```python
from build123d import *

# Parameters (mm, degrees)
CUT_EXTRUDE1_DEPTH = 20
CHAMFER1_SIZE      = 1


with BuildPart() as part:
    # Sketch1 → Revolve1 (revolve)
    with BuildSketch(Plane.XY, mode=Mode.PRIVATE) as revolve1_sk:
        Polygon((-18, 6), (18, 6), (18, 13), (5, 13), (5, 65), (13, 65), (13, 80), (-13, 80), (-13, 65), (-5, 65), (-5, 13), (-18, 13), align=None)
    revolve(revolve1_sk.sketch.rotate(Axis((0, 0, 0), (1, 0, 0)), 90), axis=Axis((0, 0, 0), (1, 0, 0)))

    # Sketch2 → Cut-Extrude1 (cut)
    with BuildSketch(Plane.ZY.offset(5)):
        with BuildLine():
            Line((-8.022576871, 61.874894191), (8.022576871, 61.874894191))
            ThreePointArc((8.022576871, 61.874894191), (11.989343573, 59.918701336), (12.852206003, 55.580798966))
            Line((12.852206003, 55.580798966), (1.931851653, 14.825481694))
            ThreePointArc((1.931851653, 14.825481694), (0, 13.343119784), (-1.931851653, 14.825481694))
            Line((-1.931851653, 14.825481694), (-12.852206003, 55.580798966))
            ThreePointArc((-12.852206003, 55.580798966), (-11.989343573, 59.918701336), (-8.022576871, 61.874894191))
        make_face()
        with BuildLine():
            Line((23.989691721, 57.596518662), (37.88520247, 49.57394179))
            ThreePointArc((37.88520247, 49.57394179), (40.342426777, 45.896445733), (38.920736376, 41.708280866))
            Line((38.920736376, 41.708280866), (9.085773454, 11.873317944))
            ThreePointArc((9.085773454, 11.873317944), (6.671559892, 11.555480699), (5.73970824, 13.805169597))
            Line((5.73970824, 13.805169597), (16.66006259, 54.560486868))
            ThreePointArc((16.66006259, 54.560486868), (19.576274559, 57.885789305), (23.989691721, 57.596518662))
        make_face()
        with BuildLine():
            Line((49.57394179, 37.88520247), (57.596518662, 23.989691721))
            ThreePointArc((57.596518662, 23.989691721), (57.885789305, 19.576274559), (54.560486868, 16.66006259))
            Line((54.560486868, 16.66006259), (13.805169597, 5.73970824))
            ThreePointArc((13.805169597, 5.73970824), (11.555480699, 6.671559892), (11.873317944, 9.085773454))
            Line((11.873317944, 9.085773454), (41.708280866, 38.920736376))
            ThreePointArc((41.708280866, 38.920736376), (45.896445733, 40.342426777), (49.57394179, 37.88520247))
        make_face()
        with BuildLine():
            Line((61.874894191, 8.022576871), (61.874894191, -8.022576871))
            ThreePointArc((61.874894191, -8.022576871), (59.918701336, -11.989343573), (55.580798966, -12.852206003))
            Line((55.580798966, -12.852206003), (14.825481694, -1.931851653))
            ThreePointArc((14.825481694, -1.931851653), (13.343119784, 0), (14.825481694, 1.931851653))
            Line((14.825481694, 1.931851653), (55.580798966, 12.852206003))
            ThreePointArc((55.580798966, 12.852206003), (59.918701336, 11.989343573), (61.874894191, 8.022576871))
        make_face()
        with BuildLine():
            Line((57.596518662, -23.989691721), (49.57394179, -37.88520247))
            ThreePointArc((49.57394179, -37.88520247), (45.896445733, -40.342426777), (41.708280866, -38.920736376))
            Line((41.708280866, -38.920736376), (11.873317944, -9.085773454))
            ThreePointArc((11.873317944, -9.085773454), (11.555480699, -6.671559892), (13.805169597, -5.73970824))
            Line((13.805169597, -5.73970824), (54.560486868, -16.66006259))
            ThreePointArc((54.560486868, -16.66006259), (57.885789305, -19.576274559), (57.596518662, -23.989691721))
        make_face()
        with BuildLine():
            Line((37.88520247, -49.57394179), (23.989691721, -57.596518662))
            ThreePointArc((23.989691721, -57.596518662), (19.576274559, -57.885789305), (16.66006259, -54.560486868))
            Line((16.66006259, -54.560486868), (5.73970824, -13.805169597))
            ThreePointArc((5.73970824, -13.805169597), (6.671559892, -11.555480699), (9.085773454, -11.873317944))
            Line((9.085773454, -11.873317944), (38.920736376, -41.708280866))
            ThreePointArc((38.920736376, -41.708280866), (40.342426777, -45.896445733), (37.88520247, -49.57394179))
        make_face()
        with BuildLine():
            Line((8.022576871, -61.874894191), (-8.022576871, -61.874894191))
            ThreePointArc((-8.022576871, -61.874894191), (-11.989343573, -59.918701336), (-12.852206003, -55.580798966))
            Line((-12.852206003, -55.580798966), (-1.931851653, -14.825481694))
            ThreePointArc((-1.931851653, -14.825481694), (0, -13.343119784), (1.931851653, -14.825481694))
            Line((1.931851653, -14.825481694), (12.852206003, -55.580798966))
            ThreePointArc((12.852206003, -55.580798966), (11.989343573, -59.918701336), (8.022576871, -61.874894191))
        make_face()
        with BuildLine():
            Line((-23.989691721, -57.596518662), (-37.88520247, -49.57394179))
            ThreePointArc((-37.88520247, -49.57394179), (-40.342426777, -45.896445733), (-38.920736376, -41.708280866))
            Line((-38.920736376, -41.708280866), (-9.085773454, -11.873317944))
            ThreePointArc((-9.085773454, -11.873317944), (-6.671559892, -11.555480699), (-5.73970824, -13.805169597))
            Line((-5.73970824, -13.805169597), (-16.66006259, -54.560486868))
            ThreePointArc((-16.66006259, -54.560486868), (-19.576274559, -57.885789305), (-23.989691721, -57.596518662))
        make_face()
        with BuildLine():
            Line((-49.57394179, -37.88520247), (-57.596518662, -23.989691721))
            ThreePointArc((-57.596518662, -23.989691721), (-57.885789305, -19.576274559), (-54.560486868, -16.66006259))
            Line((-54.560486868, -16.66006259), (-13.805169597, -5.73970824))
            ThreePointArc((-13.805169597, -5.73970824), (-11.555480699, -6.671559892), (-11.873317944, -9.085773454))
            Line((-11.873317944, -9.085773454), (-41.708280866, -38.920736376))
            ThreePointArc((-41.708280866, -38.920736376), (-45.896445733, -40.342426777), (-49.57394179, -37.88520247))
        make_face()
        with BuildLine():
            Line((-61.874894191, -8.022576871), (-61.874894191, 8.022576871))
            ThreePointArc((-61.874894191, 8.022576871), (-59.918701336, 11.989343573), (-55.580798966, 12.852206003))
            Line((-55.580798966, 12.852206003), (-14.825481694, 1.931851653))
            ThreePointArc((-14.825481694, 1.931851653), (-13.343119784, 0), (-14.825481694, -1.931851653))
            Line((-14.825481694, -1.931851653), (-55.580798966, -12.852206003))
            ThreePointArc((-55.580798966, -12.852206003), (-59.918701336, -11.989343573), (-61.874894191, -8.022576871))
        make_face()
        with BuildLine():
            Line((-57.596518662, 23.989691721), (-49.57394179, 37.88520247))
            ThreePointArc((-49.57394179, 37.88520247), (-45.896445733, 40.342426777), (-41.708280866, 38.920736376))
            Line((-41.708280866, 38.920736376), (-11.873317944, 9.085773454))
            ThreePointArc((-11.873317944, 9.085773454), (-11.555480699, 6.671559892), (-13.805169597, 5.73970824))
            Line((-13.805169597, 5.73970824), (-54.560486868, 16.66006259))
            ThreePointArc((-54.560486868, 16.66006259), (-57.885789305, 19.576274559), (-57.596518662, 23.989691721))
        make_face()
        with BuildLine():
            Line((-37.88520247, 49.57394179), (-23.989691721, 57.596518662))
            ThreePointArc((-23.989691721, 57.596518662), (-19.576274559, 57.885789305), (-16.66006259, 54.560486868))
            Line((-16.66006259, 54.560486868), (-5.73970824, 13.805169597))
            ThreePointArc((-5.73970824, 13.805169597), (-6.671559892, 11.555480699), (-9.085773454, 11.873317944))
            Line((-9.085773454, 11.873317944), (-38.920736376, 41.708280866))
            ThreePointArc((-38.920736376, 41.708280866), (-40.342426777, 45.896445733), (-37.88520247, 49.57394179))
        make_face()
    extrude(amount=-CUT_EXTRUDE1_DEPTH, mode=Mode.SUBTRACT)

    # Chamfer1
    chamfer1_edges = [part.edges().sort_by_distance(p)[0] for p in [
        (-13, 0, -65),
        (-13, 0, -80),
        (13, 0, -80),
        (13, 0, -65),
    ]]
    chamfer(chamfer1_edges, length=CHAMFER1_SIZE)


solid = part.part
```
Check sheet for the modelled part. Datum: model origin and axes. Units: mm. A direction names the side the tool comes from. Coordinates: 2 decimals unless noted, no trailing zeros. Order: outer loops, then holes, each group sorted by start corner. A loop starts at its lowest first (then second) coordinate and runs counter-clockwise, first axis right, second up. Notation, with made-up numbers: M 25,23.25 L 40,23.25 A23 cw 40,47.25 Z; hole C 15,-3 d4. An arc over 180 degrees is marked long. Write each question's results on one line, items separated by ' | '. Start each with the question number.
1. Access from +Z, -Z, +X, -X, +Y, -Y to the whole of each face (thin tool, end or side, straight path). Record for faces 1 (the face through (-0.07, -23.79, -26.58)), 2 (the face through (11.409, 7.91, -10.316)), 3 (the face through (-11.591, 7.91, -10.316)).
2. Go/stop test with flat-tipped pins: P1, Ø3, axis at x = -5.5, z = -52, coming from the -Y side; P2, Ø12, axis at y = 55.5, z = -56.5, coming from the +X side; P3, Ø8, axis at x = 7, z = 20, coming from the -Y side; P4, Ø14, axis at y = 0, z = 0, coming from the +X side. Record where each tip stops, or that it passes through.
3. Cross-section at A-A on x = -7. Record the cut outline in (y, z).
4. Mould release check, pull along Z, two halves, no side actions. Record for faces 4 (the face through (-0.07, -12.028, -59.868)), 5 (the face through (13, 64, 18)): +Z half, -Z half, draft (parallel to the pull), parting line (faces both ways), or undercut.
5. Material ranges on probe 1 along Y at (x, z) = (7, 0); probe 2 along X at (y, z) = (62.5, -4.5); probe 3 along X at (y, z) = (-5.5, 68), recorded low to high.
6. Cross-section at B-B on z = 0. State how many separate pieces and enclosed holes the cut face has, and give its area (3 significant figures).
Checks:
1) face 1: +X, -X | face 2: +X | face 3: -X
2) P1: stops at y = -62.05 | P2: stops at x = 13 | P3: stops at y = -78.38 | P4: stops at x = 18
3) outline: C 0,0 d160; C 0,0 d26; hole C 0,0 d130; hole C 0,0 d12
4) face 4: undercut | face 5: draft
5) probe 1: y = -80 to -65, -13 to -6, 6 to 13, 65 to 80 | probe 2: x = -5 to 5 | probe 3: x = -13 to 13
6) separate pieces: 4 | enclosed holes: 0 | area: 1,350 mm²
